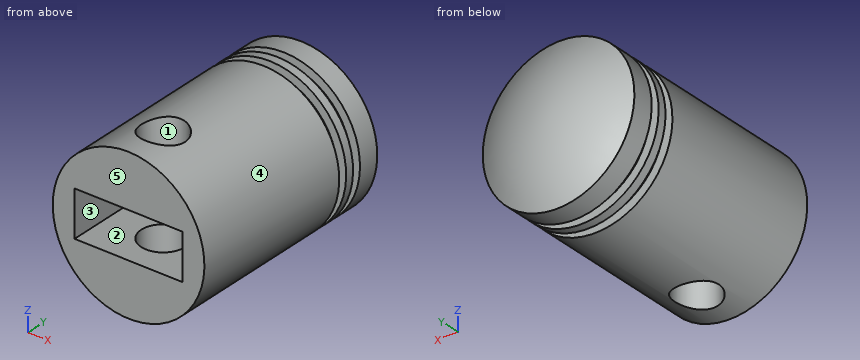
from build123d import *

# Parameters (mm, degrees)
SKETCH3_R               = 17.375
BOSS_EXTRUDE1_DEPTH     = 30
SKETCH4_R               = 17.375
BOSS_EXTRUDE2_DEPTH     = 20
CUT_EXTRUDE1_DEPTH      = 61
CUT_EXTRUDE1_DEPTH_BACK = 42
SKETCH5_R               = 5
CUT_EXTRUDE3_DEPTH      = 15
SKETCH13_W              = 24.75
SKETCH13_H              = 10.5
CUT_EXTRUDE4_DEPTH      = 9
DOME1_FACE_RADIUS       = 17.375
DOME1_HEIGHT            = 5
SKETCH16_W              = 2
SKETCH16_H              = 2


with BuildPart() as part:
    # Sketch3 → Boss-Extrude1 (new body)
    with BuildSketch(Plane(origin=(0, 0, 0), x_dir=(1, 0, 0), z_dir=(0, 1, 0))):
        with Locations(Location((0, 0, 0), (0, 0, 270))):
            Circle(SKETCH3_R)
    extrude(amount=BOSS_EXTRUDE1_DEPTH)

    # Sketch4 → Boss-Extrude2 (add)
    with BuildSketch(Plane(origin=(0, 30, 0), x_dir=(1, 0, 0), z_dir=(0, 1, 0))):
        with Locations(Location((0, 0, 0), (0, 0, 270))):
            Circle(SKETCH4_R)
    extrude(amount=BOSS_EXTRUDE2_DEPTH)

    # Sketch5 → Cut-Extrude1 (cut, two sides: drawn at the far end of the back side and taken through both)
    with BuildSketch(Plane.XY.offset(-CUT_EXTRUDE1_DEPTH_BACK)):
        with Locations(Location((0, 10, 0), (0, 0, 90.000000029))):
            Circle(SKETCH5_R)
    extrude(amount=CUT_EXTRUDE1_DEPTH + CUT_EXTRUDE1_DEPTH_BACK, mode=Mode.SUBTRACT)

    # Sketch7 → Cut-Extrude3 (cut)
    with BuildSketch(Plane.XZ):
        Polygon((0, 0), (0, 5.25), (-12.375, 5.25), (-12.375, -5.25), (0, -5.25), align=None)
        Polygon((12.375, 5.25), (0, 5.25), (0, 0), (0, -5.25), (12.375, -5.25), align=None)
    extrude(amount=-CUT_EXTRUDE3_DEPTH, mode=Mode.SUBTRACT)

    # Sketch13 → Cut-Extrude4 (cut)
    with BuildSketch(Plane.XZ.offset(-15)):
        Rectangle(SKETCH13_W, SKETCH13_H)
    extrude(amount=-CUT_EXTRUDE4_DEPTH, mode=Mode.SUBTRACT)

    # Dome1: a dome of height H over a round flat face of radius A is a cap of a sphere of radius (A * A + H * H) / (2 * H)
    dome1_r = (DOME1_FACE_RADIUS * DOME1_FACE_RADIUS + DOME1_HEIGHT * DOME1_HEIGHT) / (2 * DOME1_HEIGHT)
    dome1_base = Plane((0, 50, 0), z_dir=(0, 1, 0))
    with Locations(dome1_base.offset(DOME1_HEIGHT - dome1_r)):
        dome1_ball = Sphere(dome1_r, mode=Mode.PRIVATE)
    add(split(dome1_ball, bisect_by=dome1_base, keep=Keep.TOP, mode=Mode.PRIVATE))

    # Sketch16 → Cut-Revolve2 (revolve, cut)
    with BuildSketch(Plane.XY):
        with Locations((-16.375, 44)):
            Rectangle(SKETCH16_W, SKETCH16_H)
        with Locations((-16.375, 40)):
            Rectangle(SKETCH16_W, SKETCH16_H)
    revolve(axis=Axis((0, 55, 0), (0, -1, 0)), mode=Mode.SUBTRACT)


solid = part.part
Geometry: final body of the model. Coordinates: model frame, mm. Face numbers are marked on the shaded views. A direction names the side the tool comes from. Coordinates: 2 decimals unless noted, no trailing zeros. Loops run counter-clockwise (first coordinate to the right, second up) from the corner with the lowest first, then second, coordinate; pieces in that order, holes last. Notation, with made-up numbers: (-38, 41.25) - (-22, 41.25) arc R29 ccw to (-22, 64.25) - close; hole circle Ø5 at (23.5, 23). An arc over 180 degrees is marked (long way). One line per question, with ' | ' between items. Start each with the question number.
(1) Reachability of the marked faces 1 and 2 from +Z, -Z, +X, -X, +Y, -Y: full face, straight path, thin tool, end or side. Return the list, or none.
(2) Ray query, L1, parallel to Y at x = 13, z = -8.5; L2, parallel to Y at x = 3, z = -5.5; L3, parallel to X at y = 10, z = 14.5. Return the intervals inside material, ascending. Write a range as from..to.
(3) Draft query along Z for the marked faces 3, 4 and 5. Return one class per face: +Z half, -Z half, draft (parallel to the pull), parting line (faces both ways), or undercut.
(4) First-contact query: pin 1 (12 mm diameter, centred on y = 11.5, z = 13, fed in from -X); pin 2 (5 mm diameter, centred on x = -13, y = 45, fed in from -Z); pin 3 (1.5 mm diameter, centred on x = 5.5, y = 44.5, fed in from -Z); pin 4 (8 mm diameter, centred on x = 0, y = 10, fed in from -Z) (3 decimals). Flat tips, straight axial feed; report the tip coordinate or a pass-through.
(5) Cut plane B-B on y = 18. Output: boundary loops of the cut face in (x, z) (3 decimals).
(6) Cut plane D-D on y = 10. Output: boundary loops of the cut face in (x, z) (3 decimals), and give its area (3 significant figures).
(7) Cut plane A-A on x = 0. Count the separate pieces of the cut face and the enclosed holes in it, and give its area (3 significant figures).
(8) Cut plane C-C on z = -13. Output: boundary loops of the cut face in (x, y), and give its area (3 significant figures).
Here are the results:
1) face 1: +Z, -Z | face 2: -Y
2) L1: 0..39, 41..43, 45..51.07 | L2: 0..6, 14..54.39 | L3: -9.57..-5, 5..9.57
3) face 3: undercut | face 4: parting line | face 5: draft
4) pin 1: x = -15.9 | pin 2: z = -13.84 | pin 3: z = -16.66 | pin 4: through
5) outline: circle Ø34.75 at (0, 0); hole (-12.375, -5.25) - (12.375, -5.25) - (12.375, 5.25) - (-12.375, 5.25) - close
6) outline: (-12.375, -5.25) - (-12.375, 5.25) - (-5, 5.25) - (-5, 16.64) arc R17.375 ccw to (-5, -16.64) - (-5, -5.25) - close; (5, -16.64) arc R17.375 ccw to (5, 16.64) - (5, 5.25) - (12.375, 5.25) - (12.375, -5.25) - (5, -5.25) - close | area: 451 mm²
7) separate pieces: 3 | enclosed holes: 0 | area: 1,340 mm²
8) outline: (-11.53, 0) - (11.53, 0) - (11.53, 39) - (8.21, 39) - (8.21, 41) - (11.53, 41) - (11.53, 43) - (8.21, 43) - (8.21, 45) - (11.53, 45) - (11.53, 50) arc R29.99 ccw to (-11.53, 50) - (-11.53, 45) - (-8.21, 45) - (-8.21, 43) - (-11.53, 43) - (-11.53, 41) - (-8.21, 41) - (-8.21, 39) - (-11.53, 39) - close; hole circle Ø10 at (0, 10) | area: 1,080 mm²
